Can you work these out from the model? Positions are in its coordinate system, mm. Face numbers are marked on the shaded views. A direction names the side the tool comes from. Give positions to 0.01 mm unless a question says otherwise; leave off trailing zeros. Write each loop counter-clockwise with the first axis right and the second up, starting at its lowest first coordinate (ties: lowest second). Pieces come first, ordered by that corner, then holes. Notation, with made-up numbers: (30, -6.75) - (79, -6.75) arc R18 cw to (79, 15.25) - close; hole circle Ø1 at (-12.5, -23). An arc over 180 degrees is marked (long way). Use a Markdown table: item, result. Add a question column.
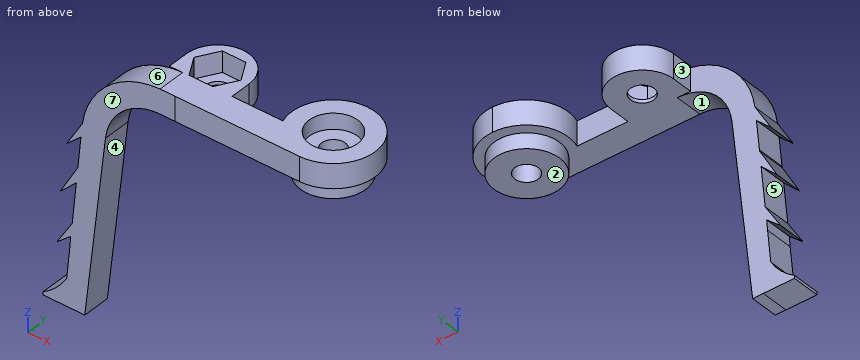
```python
from build123d import *

# Parameters (mm, degrees)
PAD022_DEPTH       = 2
PAD023_DEPTH       = 3.5
SKETCH036_R        = 3.5
POCKET003017_DEPTH = 2.25
SKETCH037_R        = 4.702209
PAD024_DEPTH       = 2.2
SKETCH038_R        = 1.7
POCKET003018_DEPTH = 5
PAD027_DEPTH       = 3.5
SKETCH044_R        = 1.7
POCKET003021_DEPTH = 5
POCKET003037_DEPTH = 3
PAD042_DEPTH       = 4


with BuildPart() as obj1:
    # Sketch034 → Pad022 (new body, symmetric)
    with BuildSketch(Plane.XZ):
        with BuildLine():
            Line((0, 28.012352), (20.118014, 28.012352))
            ThreePointArc((27.996705, 20.985645), (25.39647, 26.000475), (20.118014, 28.012352))
            Line((27.996705, 20.985645), (30.977077, -4.999855))
            Line((33.977077, -4.999855), (30.977077, -4.999855))
            Line((31.375086, 21.001563), (33.977077, -4.999855))
            ThreePointArc((31.375086, 21.001563), (27.724484, 28.375327), (20.118014, 31.512352))
            Line((0, 31.512352), (20.118014, 31.512352))
            Line((0, 28.012352), (0, 31.512352))
        make_face()
    extrude(amount=PAD022_DEPTH, both=True)

    # Sketch035 → Pad023 (new body)
    with BuildSketch(Plane(origin=(0, 0, 31.512352), x_dir=(-1, 0, 0), z_dir=(0, 0, 1))):
        with BuildLine():
            Line((-18, 2.000987), (0, 2.000987))
            ThreePointArc((2e-06, -10.000993), (6.00099, -4.000002), (0, 2.000987))
            ThreePointArc((-5.657903, -2), (-4.899687, -7.464818), (2e-06, -10.000993))
            Line((-18, -2), (-5.657903, -2))
            Line((-18, 2.000987), (-18, -2))
        make_face()
    extrude(amount=-PAD023_DEPTH)

    # Sketch036 → Pocket003017 (cut)
    with BuildSketch(Plane(origin=(0, 0, 31.512352), x_dir=(-1, 0, 0), z_dir=(0, 0, 1))):
        with Locations((0, -4)):
            Circle(SKETCH036_R)
    extrude(amount=-POCKET003017_DEPTH, mode=Mode.SUBTRACT)

    # Sketch037 → Pad024 (new body)
    with BuildSketch(Plane(origin=(0, 0, 28.012352), x_dir=(1, 0, 0), z_dir=(0, 0, -1))):
        with Locations((-0.089106, -3.841625)):
            Circle(SKETCH037_R)
    extrude(amount=PAD024_DEPTH)

    # Sketch038 → Pocket003018 (cut)
    with BuildSketch(Plane(origin=(0, 0, 25.812352), x_dir=(1, 0, 0), z_dir=(0, 0, -1))):
        with Locations((-0.080471, -3.899184)):
            Circle(SKETCH038_R)
    extrude(amount=-POCKET003018_DEPTH, mode=Mode.SUBTRACT)

    # Sketch043 → Pad027 (new body)
    with BuildSketch(Plane(origin=(0, 0, 31.512352), x_dir=(-1, 0, 0), z_dir=(0, 0, 1))):
        with BuildLine():
            Line((-22.021201, -1.987049), (-22.021201, -4.986919))
            ThreePointArc((-22.021201, -4.986919), (-17.510002, -9.511218), (-12.998803, -4.986919))
            Line((-12.998803, -4.986919), (-12.998803, -1.987049))
            Line((-22.021201, -1.987049), (-12.998803, -1.987049))
        make_face()
    extrude(amount=-PAD027_DEPTH)

    # Sketch044 → Pocket003021 (cut)
    with BuildSketch(Plane(origin=(0, 0, 31.512352), x_dir=(-1, 0, 0), z_dir=(0, 0, 1))):
        with Locations((-17.491917, -5)):
            Circle(SKETCH044_R)
    extrude(amount=-POCKET003021_DEPTH, mode=Mode.SUBTRACT)

    # Sketch071 → Pocket003037 (cut)
    with BuildSketch(Plane(origin=(0, 0, 31.512352), x_dir=(-1, 0, 0), z_dir=(0, 0, 1))):
        Polygon((-14.138998, -5.003928), (-15.835596, -2.057479), (-19.235593, -2.053552), (-20.938994, -4.996072), (-19.242396, -7.942521), (-15.842399, -7.946448), align=None)
    extrude(amount=-POCKET003037_DEPTH, mode=Mode.SUBTRACT)

    # Sketch072 → Pad042 (new body)
    with BuildSketch(Plane.XZ.offset(2)):
        with BuildLine():
            Line((27, 28.536497), (32.513573, -5))
            Line((32.513573, -5), (37.000002, -5))
            Line((37.000002, -5), (37.000002, -4.583553))
            ThreePointArc((33.505627, -1), (35.019116, -3.019659), (37.000002, -4.583553))
            Line((33, 5), (33.505627, -1))
            Line((35, 3.304739), (33, 5))
            Line((32.728943, 7), (35, 3.304739))
            Line((32, 13), (32.728943, 7))
            Line((34.496559, 10.608005), (32, 13))
            Line((32, 15), (34.496559, 10.608005))
            Line((31, 20), (32, 15))
            Line((33.606815, 17.606869), (31, 20))
            Line((31, 22), (33.606815, 17.606869))
            Line((27, 28.536497), (31, 22))
        make_face()
    extrude(amount=-PAD042_DEPTH)


with BuildPart() as part_mirroring011:
    # Part__Mirroring011: instance of obj1
    add(obj1.part.mirror(Plane(origin=(0, 0, 0), x_dir=(0, -1, 0), z_dir=(1, 0, 0))))


solid = part_mirroring011.part
```
Q1. I'm going to push flat-ended pins straight in: P1, Ø3.5, axis at x = -6, y = 6.5, coming from the -Z side; P2, Ø3, axis at x = -10.5, z = 30, coming from the +Y side; P3, Ø5, axis at y = -0.5, z = 1, coming from the -X side. Where does each tip first touch, or does it pass through?
Q2. On a 3-axis mill with a long thin cutter (end or side, diameter ignored), from which of +Z, -Z, +X, -X, +Y, -Y can I reach the whole of each face in a straight line? I mean the marked faces 1, 2 and 3. Say none if no direction works.
Q3. Suppose I cut it at B-B (x = -12). Please give me the cut outline in (y, z).
Q4. If I drill on probe 1 along Z at (x, y) = (-4.5, 0); probe 2 along Z at (x, y) = (-16, 7); probe 3 along Y at (x, z) = (-12, 28.5), over which ranges is the centre line in solid material (lowest first)? Write a range as [from, to].
Q5. If we mould it in two halves opening along X, with no side actions, what happens to the marked faces 4, 5, 6 and 7? For each: released by +X, released by -X, zero draft, split by the parting line, or undercut.
Q6. Suppose I cut it at D-D (x = -2.5). Please give me the cut outline in (y, z), and give its area (3 significant figures).
Q7. Suppose I cut it at C-C (z = -2.5). Please give me the cut outline in (x, y), and give its area (3 significant figures).
Derived:
| question | item | result |
|---|---|---|
| 1 | P1 | z = 28.01 |
| 1 | P2 | y = 2 |
| 1 | P3 | x = -35 |
| 2 | face 1 | -Z, +Y, -Y |
| 2 | face 2 | -Z, +X, +Y, -Y |
| 2 | face 3 | +Z, -Z, -X, +Y |
| 3 | outline | (-2, 28.01) - (2, 28.01) - (2, 31.51) - (-2, 31.51) - close |
| 4 | probe 1 | [28.01, 31.51] |
| 4 | probe 2 | [28.01, 28.51] |
| 4 | probe 3 | [-2, 2] |
| 5 | face 4 | released by +X |
| 5 | face 5 | undercut |
| 5 | face 6 | released by -X |
| 5 | face 7 | zero draft |
| 6 | outline | (-2, 28.01) - (-0.08, 28.01) - (-0.08, 25.81) - (7.77, 25.81) - (7.77, 28.01) - (9.46, 28.01) - (9.46, 31.51) - (6.45, 31.51) - (6.45, 29.26) - (1.55, 29.26) - (1.55, 31.51) - (-2, 31.51) - close |
| 6 | area | 46.3 mm² |
| 7 | outline | (-34.55, -2) - (-30.69, -2) - (-30.69, 2) - (-34.55, 2) - close |
| 7 | area | 15.4 mm² |
